Source: CAD feature listing. Evaluate the final solid. Frame: model axes, mm. A direction names the side the tool comes from. Give positions to 0.01 mm unless a question says otherwise; leave off trailing zeros. Order: outer loops, then holes, each group sorted by start corner. A loop starts at its lowest first (then second) coordinate and runs counter-clockwise, first axis right, second up. Notation, with made-up numbers: (21, 19) -> (27, 19) arc R21 cw to (27, 42) -> close; hole circle Ø9 at (53.5, 46). An arc over 180 degrees is marked (long way). Answer in a Markdown table with one row per item.
```python
from build123d import *

# Parameters (mm, degrees)
BOSS_EXTRUDE1_DEPTH = 1.2
BOSS_EXTRUDE3_DEPTH = 2


# Read off the part's stored shape, not the designer's step: Boss-Extrude3
with BuildPart() as part:
    # Sketch1 → Boss-Extrude1 (new body)
    with BuildSketch(Plane.XY):
        Polygon((2, 2), (29, 2), (29, -7), (31, -7), (31, -30), (0, -30), (0, -7), (2, -7), align=None)
    extrude(amount=BOSS_EXTRUDE1_DEPTH)

    # Boss-Extrude3 outline → Boss-Extrude3 (add)
    with BuildSketch(Plane(origin=(29, 0, 0), x_dir=(0, 0, -1), z_dir=(1, 0, 0))):
        with BuildLine():
            ThreePointArc((-1.2, 0.670849738), (-0.6, 0.4), (0, 0.670849738))
            Line((0, 0.670849738), (0, 1.729150262))
            ThreePointArc((0, 1.729150262), (-0.6, 2), (-1.2, 1.729150262))
            Line((-1.2, 1.729150262), (-1.2, 0.670849738))
        make_face()
    boss_extrude3 = extrude(amount=BOSS_EXTRUDE3_DEPTH)

    # Mirror1: Boss-Extrude3 across plane
    add(boss_extrude3.mirror(Plane.ZY.offset(-15.5)))


solid = part.part
```
(1) Pull-direction query (Y, two-part tool) for faces 1 (the flat face through (0, 1, 1)), 2 (the flat face through (1, -7, 1)), 3 (the cylindrical face through (1, 2, 0.6)), 4 (the flat face through (2, -3, 1)); classes: +Y half, -Y half, draft (parallel to the pull), parting line (faces both ways), or undercut.
A:
| item | result |
|---|---|
| face 1 | draft |
| face 2 | undercut |
| face 3 | +Y half |
| face 4 | undercut |
(2) First-contact query: pin 1 Ø2 at (x, y) = (15, -19) entering from -Z. Flat tip, straight axial feed; report the tip coordinate or a pass-through.
A:
| item | result |
|---|---|
| pin 1 | stops at z = 0 |
(3) Access query for faces 5 (the cylindrical face through (30, 0.4, 0.6)), 6 (the cylindrical face through (30, 2, 0.6)), 7 (the cylindrical face through (1, 0.4, 0.6)). Directions: +Z, -Z, +X, -X, +Y, -Y. A direction counts if a zero-diameter tool reaches every point of the face in a straight line with its end or side. Return the directions, or none.
A:
| item | result |
|---|---|
| face 5 | +X |
| face 6 | +X, +Y |
| face 7 | -X |
(4) Section query A-A (z = 0.25). Return the cut outline in (x, y), plus the area to 3 significant figures.
A:
| item | result |
|---|---|
| outline | (0, -30) -> (31, -30) -> (31, -7) -> (29, -7) -> (29, 0.48) -> (31, 0.48) -> (31, 1.92) -> (29, 1.92) -> (29, 2) -> (2, 2) -> (2, 1.92) -> (0, 1.92) -> (0, 0.48) -> (2, 0.48) -> (2, -7) -> (0, -7) -> close |
| area | 962 mm^2 |
(5) Ray query, probe 1 along X at (y, z) = (-3.5, 0.85). Return the intervals inside material, ascending.
A:
| item | result |
|---|---|
| probe 1 | x = 2 to 29 |
(6) Section query B-B (y = -2.5). Return the cut outline in (x, z).
A:
| item | result |
|---|---|
| outline | (2, 0) -> (29, 0) -> (29, 1.2) -> (2, 1.2) -> close |
